CAD build for the part. Positions are in the model's coordinates, mm. Face numbers are marked on the shaded views. A direction names the side the tool comes from. Round coordinates to 2 decimals unless told otherwise and drop trailing zeros. Write each loop counter-clockwise with the first axis right and the second up, starting at its lowest first coordinate (ties: lowest second). Pieces come first, ordered by that corner, then holes. Notation, with made-up numbers: (-29.5, 36.5) - (19.5, 36.5) arc R27 cw to (19.5, 61.5) - close; hole circle Ø10 at (7.25, -19). An arc over 180 degrees is marked (long way). Use one line per item in the form item = value. Start each with the question number.
Item 1: Pull direction X, two halves, no side cores. Call the marked faces 1, 2 and 3: +X half, -X half, draft (parallel to the pull), parting line (faces both ways), or undercut.
Item 2: Band-saw the part on C-C, the plane x = 18.5. List the corners of the cut face in (y, z), and give its area (3 significant figures).
Item 3: Pin check, flat tips, straight feed: pin 1 (2 mm diameter, centred on x = 23.5, y = -11, fed in from +Z); pin 2 (5.5 mm diameter, centred on x = -18.5, y = -3.75, fed in from +Z); pin 3 (13.5 mm diameter, centred on x = -1.5, z = 24, fed in from -Y); pin 4 (4 mm diameter, centred on x = -4, y = -2, fed in from -Z). Stop position of each tip, or through.
Item 4: Drill centre lines: L1, parallel to X at y = -4, z = 34; L2, parallel to Y at x = -18.5, z = 35; L3, parallel to Z at x = -0.5, y = -4. Where is each one in solid material? Low to high.
Item 5: Band-saw the part on B-B, the plane y = -3.75. List the corners of the cut face in (x, z).
Item 6: Band-saw the part on A-A, the plane z = 17.5. List the corners of the cut face in (x, y).
Item 7: Tool access for the marked faces 4 and 5: list every direction of +Z, -Z, +X, -X, +Y, -Y with a clear straight run to the whole face (end or side of a thin tool).
Item 8: Band-saw the part on D-D, the plane x = 8.5. List the corners of the cut face in (y, z).
from build123d import *

# Parameters (mm, degrees)
F0_W     = 2
F0_H     = 5
F1_DEPTH = 7.5
F3_D     = 3.4
F4_D     = 3.4
F5_DEPTH = 15


with BuildPart() as f1:
    # F0 (on Front) → F1 (new body)
    with BuildSketch(Plane.XZ):
        Polygon((-22.5, -8.5627355796), (-22.5, 34.4372644204), (22.5, 34.4372644204), (22.5, -8.5627355796), (24.5, -8.5627355796), (24.5, 36.4372644204), (-24.5, 36.4372644204), (-24.5, -8.5627355796), align=None)
        with Locations((-23.5, -11.0627355796)):
            Rectangle(F0_W, F0_H)
        with Locations((23.5, -11.0627355796)):
            Rectangle(F0_W, F0_H)
    extrude(amount=F1_DEPTH)

    # F3 (through all)
    with Locations(Plane(origin=(0, 0, 34.4372644204), x_dir=(1, 0, 0), z_dir=(0, 0, -1))):
        with Locations((-18.5, 3.75)):
            Hole(F3_D / 2)

    # F4 (through all)
    with Locations(Plane(origin=(0, 0, 34.4372644204), x_dir=(1, 0, 0), z_dir=(0, 0, -1))):
        with Locations((18.5, 3.75)):
            Hole(F4_D / 2)

    # F0 (on Front) → F5 (join)
    with BuildSketch(Plane.XZ):
        with Locations((-23.5, -11.0627355796)):
            Rectangle(F0_W, F0_H)
        with Locations((23.5, -11.0627355796)):
            Rectangle(F0_W, F0_H)
    extrude(amount=F5_DEPTH)


solid = f1.part
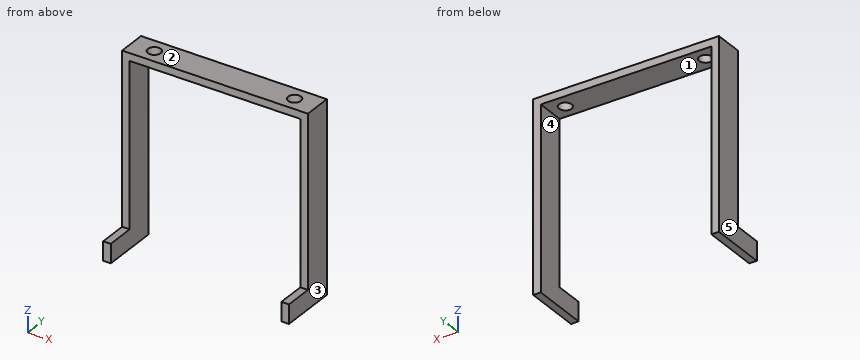
Determined:
q1.face_1 = undercut
q1.face_2 = draft
q1.face_3 = +X half
q2.outline = (-7.5, 34.44) - (-5.45, 34.44) - (-5.45, 36.44) - (-7.5, 36.44) - close; (-2.05, 34.44) - (0, 34.44) - (0, 36.44) - (-2.05, 36.44) - close
q2.area = 8.20 mm²
q3.pin_1 = -8.56
q3.pin_2 = 36.44
q3.pin_3 = through
q3.pin_4 = 34.44
q4.L1 = -24.5 to -22.5, 22.5 to 24.5
q4.L2 = -7.5 to -5.45, -2.05 to 0
q4.L3 = 34.44 to 36.44
q5.outline = (-24.5, -13.56) - (-22.5, -13.56) - (-22.5, 34.44) - (-20.2, 34.44) - (-20.2, 36.44) - (-24.5, 36.44) - close; (-16.8, 34.44) - (16.8, 34.44) - (16.8, 36.44) - (-16.8, 36.44) - close; (20.2, 34.44) - (22.5, 34.44) - (22.5, -13.56) - (24.5, -13.56) - (24.5, 36.44) - (20.2, 36.44) - close
q6.outline = (-24.5, -7.5) - (-22.5, -7.5) - (-22.5, 0) - (-24.5, 0) - close; (22.5, -7.5) - (24.5, -7.5) - (24.5, 0) - (22.5, 0) - close
q7.face_4 = -Z, +Y, -Y
q7.face_5 = +Z, -Z, -X, +Y, -Y
q8.outline = (-7.5, 34.44) - (0, 34.44) - (0, 36.44) - (-7.5, 36.44) - close
